Autodesk Inventor part; units mm, degrees
ref_plane "YZ Plane" through (0, 0, 0) normal (1, 0, 0) x (0, 1, 0)
ref_plane "XZ Plane" through (0, 0, 0) normal (0, 1, 0) x (-1, 0, 0)
ref_plane "XY Plane" through (0, 0, 0) normal (0, 0, 1) x (1, 0, 0)
sketch "Sketch1" plane through (0, 0, 0) normal (0, 1, 0) x (-1, 0, 0)
  line L0 (4.1559, 203.2) -> (4.1559, -203.2)
  line L1 (4.1559, -203.2) -> (156.5559, -291.1882)
  line L2 (4.1559, 203.2) -> (156.5559, 291.1882)
  line L3 (4.1559, 203.2) -> (180.1322, 203.2) construction
  line L4 (156.5559, 291.1882) -> (156.5559, -291.1882)
  point P0 (0, 0)
  point P1 (4.1559, 0)
  dimension "d0" = 120
  dimension "d1" = 30
  dimension "d2" = 406.4
  dimension "d5" = 152.4
extrude "Extrusion1" add sketch "Sketch1" along normal blind 6.35
sketch "Sketch3" plane through (0, 6.35, 0) normal (0, 1, 0) x (1, 0, 0)
  line L0 (-1236.8748, 812.4936) -> (-137.0225, 177.4936)
  line L1 (-1224.1748, 834.4907) -> (-1236.8748, 812.4936)
  line L2 (-124.3225, 199.4907) -> (-1224.1748, 834.4907)
  line L3 (-137.0225, 177.4936) -> (-124.3225, 199.4907)
  line L4 (-26.6836, 216.2064) -> (-1258.5181, 927.4064)
  line L5 (-39.3836, 194.2093) -> (-26.6836, 216.2064)
  line L6 (-1271.2181, 905.4093) -> (-39.3836, 194.2093)
  line L7 (-1258.5181, 927.4064) -> (-1271.2181, 905.4093)
  line L8 (-1258.5181, -927.4064) -> (-26.6836, -216.2064)
  line L9 (-1271.2181, -905.4093) -> (-1258.5181, -927.4064)
  line L10 (-39.3836, -194.2093) -> (-1271.2181, -905.4093)
  line L11 (-26.6836, -216.2064) -> (-39.3836, -194.2093)
  line L12 (-137.0225, -177.4936) -> (-1236.8748, -812.4936)
  line L13 (-124.3225, -199.4907) -> (-137.0225, -177.4936)
  line L14 (-1224.1748, -834.4907) -> (-124.3225, -199.4907)
  line L15 (-1236.8748, -812.4936) -> (-1224.1748, -834.4907)
  line L16 (-156.5559, 291.1882) -> (-156.5559, -291.1882)
  line L17 (-156.5559, -218.1006) -> (-156.5559, -188.7712)
  line L18 (-156.5559, -188.7712) -> (-137.0225, -177.4936)
  line L19 (-137.0225, -177.4936) -> (-124.3225, -199.4907)
  line L20 (-124.3225, -199.4907) -> (-156.5559, -218.1006)
  line L21 (-136.8366, -176.7997) -> (-157.0639, -188.4779)
  line L22 (-157.0639, -188.4779) -> (-157.0639, -218.9805)
  line L23 (-157.0639, -218.9805) -> (-123.6286, -199.6766)
  line L24 (-123.6286, -199.6766) -> (-136.8366, -176.7997)
  line L25 (-156.5559, -261.8588) -> (-156.5559, -291.1882)
  line L26 (-156.5559, -291.1882) -> (-26.6836, -216.2064)
  line L27 (-156.5559, -291.1882) -> (-4.1559, -203.2)
  line L28 (-26.6836, -216.2064) -> (-39.3836, -194.2093)
  line L29 (-39.3836, -194.2093) -> (-156.5559, -261.8588)
  line L30 (-157.0639, -261.5655) -> (-157.0639, -292.0681)
  line L31 (-157.0639, -292.0681) -> (-25.9896, -216.3923)
  line L32 (-25.9896, -216.3923) -> (-39.1976, -193.5154)
  line L33 (-39.1976, -193.5154) -> (-157.0639, -261.5655)
  line L34 (-156.5559, 218.1006) -> (-156.5559, 188.7712)
  line L35 (-156.5559, 188.7712) -> (-137.0225, 177.4936)
  line L36 (-137.0225, 177.4936) -> (-124.3225, 199.4907)
  line L37 (-124.3225, 199.4907) -> (-156.5559, 218.1006)
  line L38 (-157.0639, 218.9805) -> (-157.0639, 188.4779)
  line L39 (-157.0639, 188.4779) -> (-136.8366, 176.7997)
  line L40 (-136.8366, 176.7997) -> (-123.6286, 199.6766)
  line L41 (-123.6286, 199.6766) -> (-157.0639, 218.9805)
  line L42 (-156.5559, 261.8588) -> (-156.5559, 291.1882)
  line L43 (-156.5559, 291.1882) -> (-26.6836, 216.2064)
  line L44 (-26.6836, 216.2064) -> (-39.3836, 194.2093)
  line L45 (-39.3836, 194.2093) -> (-156.5559, 261.8588)
  line L46 (-157.0639, 261.5655) -> (-157.0639, 292.0681)
  line L47 (-157.0639, 292.0681) -> (-25.9896, 216.3923)
  line L48 (-25.9896, 216.3923) -> (-39.1976, 193.5154)
  line L49 (-39.1976, 193.5154) -> (-157.0639, 261.5655)
  point P0 (0, 0)
  dimension "d6" = 0.508
  dimension "d7" = 0.508
  dimension "d8" = 0.508
  dimension "d9" = 0.508
extrude "Extrusion2" cut sketch "Sketch3" against normal through all contours L16 L2 L3 L0 | L16 L39 L38 L0 | L0 L38 L2 L16 | L0 L3 L2 L16 L41 L40 L39 | L49 L46 L6 L16 | L16 L6 L5 L4 L46 L47 L48 L49 | L33 L32 L27 L11 L10 L16 | L16 L10 L30 L33 | L21 L24 L23 L16 L14 L13 L12 | L16 L12 L22 L21 | L0 L1 L2 L38 | L2 L38 L41 L16 | L16 L14 L22 L12 | L12 L13 L14 L16 | L16 L4 L5 L6 | L6 L46 L4 L16 | L22 L14 L15 L12 | L16 L23 L22 L14 | L16 L8 L30 L10 | L10 L11 L8 L16 | L8 L27 L32 L31 L30
sketch "Sketch4" plane through (0, 6.35, 0) normal (0, 1, 0) x (1, 0, 0)
  line L0 (-4.1559, -203.2) -> (-4.1559, 203.2)
  point P0 (0, 0)
  point P1 (-80.3559, 0)
  dimension "d12" = 76.2
  dimension "d13" = 203.2
hole "Hole1" at (-80.3559, 6.35, 0) direction (0, -1, 0) diameter 13.4925 end through all
properties part number "Triangle End"
Geometry: final body of the model. Coordinates: model frame, mm. A direction names the side the tool comes from. Round coordinates to 2 decimals unless told otherwise and drop trailing zeros. Order: outer loops, then holes, each group sorted by start corner. A loop starts at its lowest first (then second) coordinate and runs counter-clockwise, first axis right, second up. Notation, with made-up numbers: (-11.75, 30) -> (40.25, 30) arc R19 cw to (40.25, 39) -> close; hole circle Ø5 at (6, 22). An arc over 180 degrees is marked (long way). Use one line per item in the form item = value.
(1) First-contact query: pin 1 Ø1 at (y, z) = (3, -203) entering from -X; pin 2 Ø1 at (x, y) = (-64, 3) entering from +Z; pin 3 Ø1 at (x, y) = (-58, 4.5) entering from -Z. Flat tips, straight axial feed; report the tip coordinate or a pass-through.
Results list:
pin_1 = -130.25
pin_2 = 208.12
pin_3 = -204.66
(2) Section A-A on z = 0. Return loops of the section in (x, y).
Results list:
outline = (-156.56, 0) -> (-87.1, 0) -> (-87.1, 6.35) -> (-156.56, 6.35) -> close; (-73.61, 0) -> (-4.16, 0) -> (-4.16, 6.35) -> (-73.61, 6.35) -> close
(3) Access query for faces 1 (the face through (-140.3, 3.2, 209.3)), 2 (the face through (-97.06, 3.22, 226.92)), 3 (the face through (-146.83, 3.22, -182.57)), 4 (the face through (-32.63, 3.22, -204.89)). Directions: +Z, -Z, +X, -X, +Y, -Y. A direction counts if a zero-diameter tool reaches every point of the face in a straight line with its end or side. Return the directions, or none.
Results list:
face_1 = -X, +Y, -Y
face_2 = +Z, +Y, -Y
face_3 = +Y, -Y
face_4 = -Z, +Y, -Y
(4) Ray query, probe 1 along X at (y, z) = (3.75, 0); probe 2 along Z at (x, y) = (-76.5, 4.5); probe 3 along Z at (x, y) = (-134, 1). Return the intervals inside material, ascending. Write a range as [from, to].
Results list:
probe_1 = [-156.56, -87.1], [-73.61, -4.16]
probe_2 = [-215.05, -5.54], [5.54, 215.05]
probe_3 = [-248.25, -205.66], [-181.71, 181.71], [205.66, 248.25]
(5) Section B-B on y = 2.25. Return loops of the section in (x, z).
Results list:
outline = (-156.56, -261.27) -> (-39.2, -193.52) -> (-26.24, -215.95) -> (-4.16, -203.2) -> (-4.16, 203.2) -> (-26.24, 215.95) -> (-39.2, 193.52) -> (-156.56, 261.27) -> (-156.56, 218.69) -> (-123.63, 199.68) -> (-136.84, 176.8) -> (-156.56, 188.18) -> (-156.56, -188.18) -> (-136.84, -176.8) -> (-123.63, -199.68) -> (-156.56, -218.69) -> close; hole circle Ø13.49 at (-80.36, 0)
(6) Section C-C on x = -114.5. Return loops of the section in (y, z), and give its area (3 significant figures).
Results list:
outline = (0, -236.99) -> (6.35, -236.99) -> (6.35, 236.99) -> (0, 236.99) -> close
area = 3,010 mm^2
(7) Draft query along X for faces 5 (the face through (-139.86, 3.22, -209.05)), 6 (the face through (-130.325, 3.219, -188.078)), 7 (the face through (-15.05, 3.13, -209.49)). Return one class per face: pulls with the +X half, pulls with the -X half, needs draft (parallel to the pull), parting line crosses it, or undercut.
Results list:
face_5 = pulls with the -X half
face_6 = undercut
face_7 = pulls with the +X half
